from build123d import *

# Parameters (mm, degrees)
ESQUISSE1_R        = 10.5
ESQUISSE1_R_2      = 2.5
BOSS_EXTRU_1_DEPTH = 1
ESQUISSE2_R        = 8.75
ESQUISSE2_R_2      = 2.5
BOSS_EXTRU_2_DEPTH = 10
ESQUISSE3_R        = 10.5
ESQUISSE3_R_2      = 2.5
BOSS_EXTRU_3_DEPTH = 1


with BuildPart() as part:
    # Esquisse1 → Boss.-Extru.1 (new body)
    with BuildSketch(Plane.XY):
        Circle(ESQUISSE1_R)
        Circle(ESQUISSE1_R_2, mode=Mode.SUBTRACT)
    extrude(amount=BOSS_EXTRU_1_DEPTH)

    # Esquisse2 → Boss.-Extru.2 (add)
    with BuildSketch(Plane(origin=(0, 0, 0), x_dir=(-1, 0, 0), z_dir=(0, 0, -1))):
        Circle(ESQUISSE2_R)
        Circle(ESQUISSE2_R_2, mode=Mode.SUBTRACT)
    extrude(amount=BOSS_EXTRU_2_DEPTH)

    # Esquisse3 → Boss.-Extru.3 (add)
    with BuildSketch(Plane(origin=(0, 0, -10), x_dir=(-1, 0, 0), z_dir=(0, 0, -1))):
        Circle(ESQUISSE3_R)
        Circle(ESQUISSE3_R_2, mode=Mode.SUBTRACT)
    extrude(amount=BOSS_EXTRU_3_DEPTH)


solid = part.part
Could you check a few things on this model? Use its own coordinates, in mm. A direction names the side the tool comes from. Give positions to 0.01 mm unless a question says otherwise; leave off trailing zeros. Order: outer loops, then holes, each group sorted by start corner. A loop starts at its lowest first (then second) coordinate and runs counter-clockwise, first axis right, second up.
1. Suppose I cut it at C-C (z = -2.5). Write out the boundary of the cut face in (x, y).
Answers below:
outline: circle Ø17.5 at (0, 0); hole circle Ø5 at (0, 0)
2. For pin 1 (1 mm diameter, centred on x = -3.5, z = -4, fed in from +Y); pin 2 (3 mm diameter, centred on x = 2, z = -0.5, fed in from -Y); pin 3 (5 mm diameter, centred on x = -7, z = -6, fed in from +Y), each with a flat end and sliding along its axis, tell me the tip position at first contact or that it passes through.
Answers below:
pin 1: stops at y = 8.22
pin 2: stops at y = -10.48
pin 3: stops at y = 7.5
3. I need wall thicknesses on L1, parallel to Z at x = 8.25, y = -5; L2, parallel to Y at x = 0, z = 0.55; L3, parallel to Y at x = 1.5, z = -5.25. Which ranges of each line are inside material? Lowest first, please.
Answers below:
L1: z = -11 to -10, 0 to 1
L2: y = -10.5 to -2.5, 2.5 to 10.5
L3: y = -8.62 to -2, 2 to 8.62
4. Thinking about a two-plate mould opening in Z: for faces 3 (the cylindrical face through (-10, 3.2, -10.5)), 4 (the flat face through (-2, -2, -11)), 5 (the flat face through (2, -2, 1)), 6 (the flat face through (-4, 8, 0)), which applies, +Z half, -Z half, draft (parallel to the pull), parting line (faces both ways), or undercut?
Answers below:
face 3: draft
face 4: -Z half
face 5: +Z half
face 6: undercut
5. Suppose I cut it at D-D (y = 4.25). Write out the boundary of the cut face in (x, z).
Answers below:
outline: (-9.6, -11) - (9.6, -11) - (9.6, -10) - (7.65, -10) - (7.65, 0) - (9.6, 0) - (9.6, 1) - (-9.6, 1) - (-9.6, 0) - (-7.65, 0) - (-7.65, -10) - (-9.6, -10) - close
6. Which directions (+Z, -Z, +X, -X, +Y, -Y) give clear straight access to the entire face, cutting with the end or side of a thin tool? Please do faces 1 (the flat face through (4, 8, -10)), 2 (the cylindrical face through (10, 3.2, 0.5)).
Answers below:
face 1: none
face 2: +Z, -Z
7. Suppose I cut it at A-A (x = 0). Write out the boundary of the cut face in (y, z).
Answers below:
outline: (-10.5, -11) - (-2.5, -11) - (-2.5, 1) - (-10.5, 1) - (-10.5, 0) - (-8.75, 0) - (-8.75, -10) - (-10.5, -10) - close; (2.5, -11) - (10.5, -11) - (10.5, -10) - (8.75, -10) - (8.75, 0) - (10.5, 0) - (10.5, 1) - (2.5, 1) - close
